Design review of the part shown in the three views and the two pictorial views. Dimensions are in mm from the part's minimum x, y and z. A direction names the side the tool comes from. Round coordinates to 2 decimals unless told otherwise and drop trailing zeros. Loops run counter-clockwise (first coordinate to the right, second up) from the corner with the lowest first, then second, coordinate; pieces in that order, holes last. Notation, with made-up numbers: (-1.5, 27.25) - (44.5, 27.25) arc R23 cw to (44.5, 60.25) - close; hole circle Ø11 at (58.25, 16). An arc over 180 degrees is marked (long way). Return JSON: item names as keys, results as strings. Group by question number.
(1) We need section D-D, the plane z = 2.5. Write out the cut boundary in (x, y), and give its area (3 significant figures).
(2) Clearance check with flat-ended pins moving along their axes: pin 1 (10 mm diameter, centred on x = 40.5, z = 17.5, fed in from +Y); pin 2 (3 mm diameter, centred on y = 5, z = 19.5, fed in from +X). State where each tip first meets the part, or that it passes through.
(3) For the marked faces 1 and 2, list the 3-axis set-ups (+Z, -Z, +X, -X, +Y, -Y) from which the entire face can be reached by the end or side of a thin tool; tool diameter is ignored.
(4) We need section C-C, the plane x = 4.2. Write out the cut boundary in (y, z) (1 decimal), and give its area (3 significant figures).
(5) We need section A-A, the plane z = 20. Write out the cut boundary in (x, y).
(6) We need section B-B, the plane y = 2.75. Write out the cut boundary in (x, z) (1 decimal).
(7) Wall thickness on L1, parallel to Y at x = 4, z = 21; L2, parallel to X at y = 4.2, z = 24.5; L3, parallel to X at y = 2.5, z = 7.5: over which ranges is each line inside the solid? List them lowest first. Write a range as [from, to].
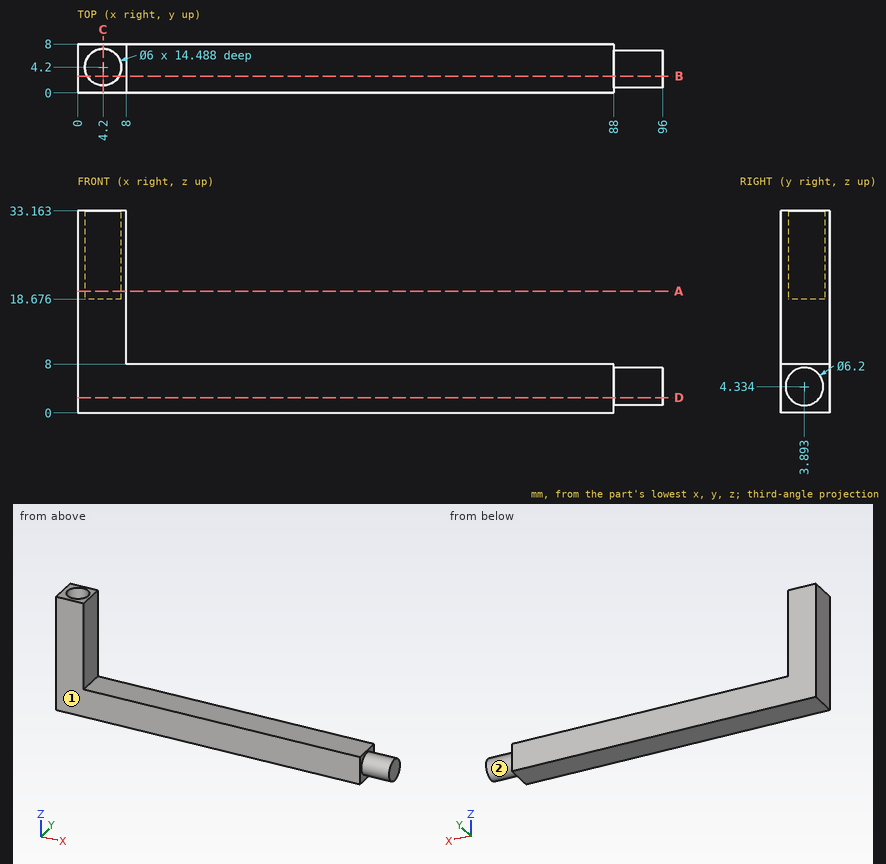
Solutions:
{
 "1": {"outline": "(0, 0) - (88, 0) - (88, 1.39) - (96, 1.39) - (96, 6.39) - (88, 6.39) - (88, 8) - (0, 8) - close", "area": "744 mm^2"},
 "2": {"pin 1": "through", "pin 2": "x = 8"},
 "3": {"face 1": "+Z, -Z, +X, -X, -Y", "face 2": "+X"},
 "4": {"outline": "(0, 0) - (8, 0) - (8, 33.2) - (7.2, 33.2) - (7.2, 18.7) - (1.2, 18.7) - (1.2, 33.2) - (0, 33.2) - close", "area": "178 mm^2"},
 "5": {"outline": "(0, 0) - (8, 0) - (8, 8) - (0, 8) - close; hole circle Ø6 at (4.2, 4.2)"},
 "6": {"outline": "(0, 0) - (88, 0) - (88, 1.5) - (96, 1.5) - (96, 7.2) - (88, 7.2) - (88, 8) - (8, 8) - (8, 33.2) - (6.8, 33.2) - (6.8, 18.7) - (1.6, 18.7) - (1.6, 33.2) - (0, 33.2) - close"},
 "7": {"L1": "[0, 1.21], [7.19, 8]", "L2": "[0, 1.2], [7.2, 8]", "L3": "[0, 88]"}
}
